```python
from build123d import *

# Parameters (mm, degrees)
SKETCH009_W      = 32
SKETCH009_H      = 32
EXTRUDE009_DEPTH = 3
SKETCH005_R      = 2.1
EXTRUDE007_DEPTH = 4
SKETCH008_R      = 4
EXTRUDE008_DEPTH = 5
CYLINDER_R       = 7
CYLINDER_DEPTH   = 1.5
EXTRUDE006_DEPTH = 2
SKETCH012_R      = 0.95
EXTRUDE011_DEPTH = 7
SKETCH013_R      = 2.1
SKETCH013_R_2    = 1.25
EXTRUDE012_DEPTH = 27.5
EXTRUDE005_DEPTH = 20


with BuildPart() as cone004:
    # Cone004 → Cone004 (revolve)
    with BuildSketch(Plane(origin=(-13, -9, -19.9), x_dir=(-1, 0, 0), z_dir=(0, 1, 0))):
        Polygon((0, 0), (2.1, 0), (6, 20), (0, 20), align=None)
    revolve(axis=Axis((-13, -9, -19.9), (0, 0, 1)))


with BuildPart() as cone005:
    # Cone005 → Cone005 (revolve)
    with BuildSketch(Plane(origin=(-13, -58, -19.8), x_dir=(-1, 0, 0), z_dir=(0, 1, 0))):
        Polygon((0, 0), (2.1, 0), (6, 20), (0, 20), align=None)
    revolve(axis=Axis((-13, -58, -19.8), (0, 0, 1)))


with BuildPart() as cone006:
    # Cone006 → Cone006 (revolve)
    with BuildSketch(Plane(origin=(-71, -9, -19.9), x_dir=(1, 0, 0), z_dir=(0, -1, 0))):
        Polygon((0, 0), (2.1, 0), (6, 20), (0, 20), align=None)
    revolve(axis=Axis((-71, -9, -19.9), (0, 0, 1)))


with BuildPart() as cone007:
    # Cone007 → Cone007 (revolve)
    with BuildSketch(Plane(origin=(-71, -58, -19.7), x_dir=(1, 0, 0), z_dir=(0, -1, 0))):
        Polygon((0, 0), (2.1, 0), (6, 20), (0, 20), align=None)
    revolve(axis=Axis((-71, -58, -19.7), (0, 0, 1)))


with BuildPart() as extrude009:
    # Sketch009 (on Face3 of Fusion001) → Extrude009 (new body)
    with BuildSketch(Plane.XZ.offset(100)):
        with Locations((-30, -29)):
            Rectangle(SKETCH009_W, SKETCH009_H)
    extrude(amount=-EXTRUDE009_DEPTH)


with BuildPart() as extrude007:
    # Sketch005 → Extrude007 (new body)
    with BuildSketch(Plane.XY):
        with Locations((-62.5, -27.5)):
            Circle(SKETCH005_R)
        with Locations((-41.5, -27.5)):
            Circle(SKETCH005_R)
        with Locations((-41.5, -40)):
            Circle(SKETCH005_R)
        with Locations((-62.5, -40)):
            Circle(SKETCH005_R)
    extrude(amount=-EXTRUDE007_DEPTH)


with BuildPart() as extrude008:
    # Sketch008 → Extrude008 (new body, symmetric)
    with BuildSketch(Plane.XY):
        with Locations((-52, -40)):
            Circle(SKETCH008_R)
    extrude(amount=EXTRUDE008_DEPTH, both=True)


with BuildPart() as cylinder:
    # Cylinder → Cylinder (new body)
    with BuildSketch(Plane(origin=(-52, -40.15, 0.25), x_dir=(1, 0, 0), z_dir=(0, 0, -1))):
        Circle(CYLINDER_R)
    extrude(amount=CYLINDER_DEPTH)


with BuildPart() as cut002:
    # Sketch007 → Extrude006 (new body)
    with BuildSketch(Plane.XY):
        Polygon((0, 0), (0, -100), (-54, -100), (-104, -86), (-104, 0), align=None)
    extrude(amount=EXTRUDE006_DEPTH)

    # Fusion005: union Cylinder
    add(cylinder.part)

    # Cut002: cut Extrude008
    add(extrude008.part, mode=Mode.SUBTRACT)


with BuildPart() as extrude011:
    # Sketch012 → Extrude011 (new body)
    with BuildSketch(Plane.XY):
        with Locations((-62.5, -27.5)):
            Circle(SKETCH012_R)
        with Locations((-41.5, -27.5)):
            Circle(SKETCH012_R)
        with Locations((-41.5, -40)):
            Circle(SKETCH012_R)
        with Locations((-62.5, -40)):
            Circle(SKETCH012_R)
    extrude(amount=-EXTRUDE011_DEPTH)


with BuildPart() as extrude012:
    # Sketch013 → Extrude012 (new body)
    with BuildSketch(Plane.XY):
        with Locations((-71, -9)):
            Circle(SKETCH013_R)
        with Locations((-71, -9)):
            Circle(SKETCH013_R_2, mode=Mode.SUBTRACT)
        with Locations((-13, -9)):
            Circle(SKETCH013_R)
        with Locations((-13, -9)):
            Circle(SKETCH013_R_2, mode=Mode.SUBTRACT)
        with Locations((-13, -58)):
            Circle(SKETCH013_R)
        with Locations((-13, -58)):
            Circle(SKETCH013_R_2, mode=Mode.SUBTRACT)
        with Locations((-71, -58)):
            Circle(SKETCH013_R)
        with Locations((-71, -58)):
            Circle(SKETCH013_R_2, mode=Mode.SUBTRACT)
    extrude(amount=-EXTRUDE012_DEPTH)


with BuildPart() as fusion004:
    # Sketch006 → Extrude005 (new body)
    with BuildSketch(Plane.XY):
        Polygon((0, 0), (0, -100), (-54, -100), (-104, -86), (-104, 0), align=None)
        Polygon((-3, -3), (-3, -97), (-54, -97), (-101, -83.84), (-101, -3), align=None, mode=Mode.SUBTRACT)
    extrude(amount=-EXTRUDE005_DEPTH)

    # Fusion001: union Extrude007, Cut002, Extrude011, Extrude012
    add(extrude007.part)
    add(cut002.part)
    add(extrude011.part)
    add(extrude012.part)

    # Cut003: cut Extrude009
    add(extrude009.part, mode=Mode.SUBTRACT)

    # Fusion004: union Cone004, Cone005, Cone006, Cone007
    add(cone004.part)
    add(cone005.part)
    add(cone006.part)
    add(cone007.part)


solid = fusion004.part
```
Verification items for the finished model (mm, model axes). A direction names the side the tool comes from. Round coordinates to 2 decimals unless told otherwise and drop trailing zeros. Order: outer loops, then holes, each group sorted by start corner. A loop starts at its lowest first (then second) coordinate and runs counter-clockwise, first axis right, second up. Notation, with made-up numbers: (-33.75, 23) - (21.25, 23) arc R28 ccw to (21.25, 48) - close; hole circle Ø10 at (33.25, -4). An arc over 180 degrees is marked (long way). Use CSV: the item, a comma, the result in double quotes.
(1) Gauge pin test, flat ends, axial feed: pin 1 Ø6 at (y, z) = (-38.5, -11.5) entering from +X; pin 2 Ø3.5 at (x, y) = (-62.5, -40) entering from -Z; pin 3 Ø0.8 at (x, y) = (-13, -58.5) entering from -Z; pin 4 Ø3 at (x, y) = (-35, -20.5) entering from -Z. Record the tip position at first contact, or that the pin passes through.
Entries:
pin 1,"x = 0"
pin 2,"z = -7"
pin 3,"z = -19.8"
pin 4,"z = 0"
(2) Section check B-B on x = -52. Record the boundary of the cut face in (y, z), and give its area (4 significant figures).
Entries:
outline,"(-100, -20) - (-97, -20) - (-97, 0) - (-47.15, 0) - (-47.15, -1.25) - (-44, -1.25) - (-44, 2) - (-100, 2) - close; (-36, -1.25) - (-33.15, -1.25) - (-33.15, 0) - (-3, 0) - (-3, -20) - (0, -20) - (0, 2) - (-36, 2) - close"
area,"311.5 mm^2"
(3) Section check C-C on y = -58. Record the boundary of the cut face in (x, z), and give its area (3 significant figures).
Entries:
outline,"(-104, -20) - (-101, -20) - (-101, 0) - (-76.94, 0) - (-73.1, -19.7) - (-73.1, -27.5) - (-72.25, -27.5) - (-72.25, -19.7) - (-69.75, -19.7) - (-69.75, -27.5) - (-68.9, -27.5) - (-68.9, -19.7) - (-65.06, 0) - (-18.96, 0) - (-15.1, -19.8) - (-15.1, -27.5) - (-14.25, -27.5) - (-14.25, -19.8) - (-11.75, -19.8) - (-11.75, -27.5) - (-10.9, -27.5) - (-10.9, -19.8) - (-7.04, 0) - (-3, 0) - (-3, -20) - (0, -20) - (0, 2) - (-104, 2) - close"
area,"672 mm^2"
(4) Access from +Z, -Z, +X, -X, +Y, -Y to the whole of each face (thin tool, end or side, straight path). Record for faces 1 (the face through (-70, -10, -27.5)), 2 (the face through (-3, -49, -10)).
Entries:
face 1,"-Z, +X, -X, +Y, -Y"
face 2,"-Z"
(5) Mould release check, pull along Y, two halves, no side actions. Record for faces 3 (the face through (-49, -37, -1.25)), 4 (the face through (-12, -59, -27.5)), 5 (the face through (-75.044, -57.822, -9.712)): released by +Y, released by -Y, zero draft, split by the parting line, or undercut.
Entries:
face 3,"undercut"
face 4,"zero draft"
face 5,"undercut"
(6) Thickness scan on probe 1 along Y at (x, z) = (-71, -21.75); probe 2 along X at (y, z) = (-19, -16.25); probe 3 along Z at (x, y) = (-93, -68.5). Record the ranges inside material, lowest first. Write a range as from..to.
Entries:
probe 1,"-60.1..-59.25, -56.75..-55.9, -11.1..-10.25, -7.75..-6.9"
probe 2,"-104..-101, -3..0"
probe 3,"0..2"
(7) Section check A-A on z = -11.25. Record the boundary of the cut face in (x, y).
Entries:
outline,"(-104, -86) - (-54, -100) - (0, -100) - (0, 0) - (-104, 0) - close; circle Ø7.57 at (-71, -9); circle Ø7.5 at (-71, -58); circle Ø7.57 at (-13, -9); circle Ø7.53 at (-13, -58); hole (-101, -83.84) - (-54, -97) - (-3, -97) - (-3, -3) - (-101, -3) - close"
